Input: part model. Units: mm. Frame: model coordinates. Give positions to 0.01 mm unless a question says otherwise; leave off trailing zeros. Write each loop counter-clockwise with the first axis right and the second up, starting at its lowest first coordinate (ties: lowest second). Pieces come first, ordered by that corner, then holes. Notation, with made-up numbers: (88, 33.25) -> (98, 33.25) arc R35 ccw to (98, 72.25) -> close; hole circle Ø11 at (-23.75, 87). An arc over 180 degrees is marked (long way). Return JSON: item names as keys, results as strings. Group by question number.
Item 1: Pin query (flat end, axial travel): P1, Ø2, axis at y = 26.5, z = 5.5, coming from the +X side; P2, Ø3.5, axis at x = -30, y = -11.25, coming from the -Z side; P3, Ø2.5, axis at x = 110, y = 18.63, coming from the -Z side; P4, Ø5, axis at x = 20, y = -11.25, coming from the +Z side. Return the tip coordinate at first contact, or that it passes through.
Item 2: Section A-A, the plane x = -71. Return loops of the section in (y, z).
Item 3: Line query: line 1 (Y direction, x = 110, z = 2.5); line 2 (Y direction, x = 25, z = 2.3); line 3 (Y direction, x = -30, z = 1.35). Output: solid intervals per line, ascending. Write a range as [from, to].
from build123d import *

# Parameters (mm, degrees)
SKETCH_1_R      = 1.55
SKETCH_1_R_2    = 1.6
SKETCH_1_R_3    = 1.546583653
SKETCH_1_R_4    = 2
EXTRUDE_1_DEPTH = 4
EXTRUDE_2_DEPTH = 2


with BuildPart() as part:
    # 草图1 → 凸台-拉伸1 (new body)
    with BuildSketch(Plane.XY):
        with BuildLine():
            Line((-93.257786629, 4.43161967), (-67.403754616, 4.43161967))
            ThreePointArc((-67.403754616, 4.43161967), (-63.86822071, 2.967153575), (-62.403754616, -0.56838033))
            Line((-62.403754616, -0.56838033), (-62.403754616, -2.789641507))
            ThreePointArc((-62.403754616, -2.789641507), (-58.770779001, -11.560420508), (-50, -15.193396123))
            Line((-50, -15.193396123), (-25.75, -15.193396123))
            ThreePointArc((-25.75, -15.193396123), (-18.678932188, -18.122328311), (-15.75, -25.193396123))
            Line((-15.75, -25.193396123), (-15.75, -53.504719017))
            Line((-15.75, -53.504719017), (15.75, -53.504719017))
            Line((15.75, -53.504719017), (15.75, -25.193396123))
            ThreePointArc((15.75, -25.193396123), (18.678932188, -18.122328311), (25.75, -15.193396123))
            Line((25.75, -15.193396123), (50, -15.193396123))
            ThreePointArc((50, -15.193396123), (58.770779001, -11.560420508), (62.403754616, -2.789641507))
            Line((62.403754616, -2.789641507), (62.403754616, -0.56838033))
            ThreePointArc((62.403754616, -0.56838033), (63.86822071, 2.967153575), (67.403754616, 4.43161967))
            Line((67.403754616, 4.43161967), (93.257786629, 4.43161967))
            Line((93.257786629, 4.43161967), (115, 4.43161967))
            ThreePointArc((115, 4.43161967), (122.071067812, 7.360551858), (125, 14.43161967))
            Line((125, 14.43161967), (125, 44.220324858))
            ThreePointArc((125, 44.220324858), (122.071067812, 51.29139267), (115, 54.220324858))
            Line((115, 54.220324858), (95.550812853, 54.220324858))
            Line((95.550812853, 54.220324858), (-95.550812853, 54.220324858))
            Line((-95.550812853, 54.220324858), (-115, 54.220324858))
            ThreePointArc((-115, 54.220324858), (-122.071067812, 51.29139267), (-125, 44.220324858))
            Line((-125, 44.220324858), (-125, 14.43161967))
            ThreePointArc((-125, 14.43161967), (-122.071067812, 7.360551858), (-115, 4.43161967))
            Line((-115, 4.43161967), (-93.257786629, 4.43161967))
        make_face()
        with Locations((-10.5, -32.252284296)):
            Circle(SKETCH_1_R, mode=Mode.SUBTRACT)
        with Locations((-49, -5.252284296)):
            Circle(SKETCH_1_R, mode=Mode.SUBTRACT)
        with Locations((-30, -11.252284296)):
            Circle(SKETCH_1_R, mode=Mode.SUBTRACT)
        with Locations((-20, -11.252284296)):
            Circle(SKETCH_1_R, mode=Mode.SUBTRACT)
        with Locations((-10.5, -11.252284296)):
            Circle(SKETCH_1_R, mode=Mode.SUBTRACT)
        with Locations((-25, -0.752284296)):
            Circle(SKETCH_1_R, mode=Mode.SUBTRACT)
        with Locations((0, -42.752284296)):
            Circle(SKETCH_1_R_2, mode=Mode.SUBTRACT)
        with Locations((10.5, -32.252284296)):
            Circle(SKETCH_1_R, mode=Mode.SUBTRACT)
        with Locations((0, -21.748867949)):
            Circle(SKETCH_1_R_3, mode=Mode.SUBTRACT)
        with Locations((10.5, -11.252284296)):
            Circle(SKETCH_1_R, mode=Mode.SUBTRACT)
        with Locations((20, -11.252284296)):
            Circle(SKETCH_1_R, mode=Mode.SUBTRACT)
        with Locations((30, -11.252284296)):
            Circle(SKETCH_1_R, mode=Mode.SUBTRACT)
        with Locations((0, -0.752284296)):
            Circle(SKETCH_1_R, mode=Mode.SUBTRACT)
        with Locations((25, -0.752284296)):
            Circle(SKETCH_1_R, mode=Mode.SUBTRACT)
        with Locations((49, -5.252284296)):
            Circle(SKETCH_1_R, mode=Mode.SUBTRACT)
        with Locations((-110, 18.626388225)):
            Circle(SKETCH_1_R_4, mode=Mode.SUBTRACT)
        with BuildLine():
            ThreePointArc((-47.619318323, 12.788573549), (-49.619318323, 14.788573549), (-47.619318323, 16.788573549))
            Line((-47.619318323, 16.788573549), (-22.619318323, 16.788573549))
            ThreePointArc((-22.619318323, 16.788573549), (-20.619318323, 14.788573549), (-22.619318323, 12.788573549))
            Line((-22.619318323, 12.788573549), (-47.619318323, 12.788573549))
        make_face(mode=Mode.SUBTRACT)
        with Locations((-120.5, 29.126388225)):
            Circle(SKETCH_1_R_4, mode=Mode.SUBTRACT)
        with Locations((-99.5, 29.126388225)):
            Circle(SKETCH_1_R_4, mode=Mode.SUBTRACT)
        with Locations((-110, 39.626388225)):
            Circle(SKETCH_1_R_4, mode=Mode.SUBTRACT)
        with BuildLine():
            ThreePointArc((-47.619318323, 32.223901574), (-49.619318323, 34.223901574), (-47.619318323, 36.223901574))
            Line((-47.619318323, 36.223901574), (-22.619318323, 36.223901574))
            ThreePointArc((-22.619318323, 36.223901574), (-20.619318323, 34.223901574), (-22.619318323, 32.223901574))
            Line((-22.619318323, 32.223901574), (-47.619318323, 32.223901574))
        make_face(mode=Mode.SUBTRACT)
        with BuildLine():
            Line((22.619318323, 16.788573549), (47.619318323, 16.788573549))
            ThreePointArc((47.619318323, 16.788573549), (49.619318323, 14.788573549), (47.619318323, 12.788573549))
            Line((47.619318323, 12.788573549), (22.619318323, 12.788573549))
            ThreePointArc((22.619318323, 12.788573549), (20.619318323, 14.788573549), (22.619318323, 16.788573549))
        make_face(mode=Mode.SUBTRACT)
        with Locations((110, 18.626388225)):
            Circle(SKETCH_1_R_4, mode=Mode.SUBTRACT)
        with BuildLine():
            Line((22.619318323, 36.223901574), (47.619318323, 36.223901574))
            ThreePointArc((47.619318323, 36.223901574), (49.619318323, 34.223901574), (47.619318323, 32.223901574))
            Line((47.619318323, 32.223901574), (22.619318323, 32.223901574))
            ThreePointArc((22.619318323, 32.223901574), (20.619318323, 34.223901574), (22.619318323, 36.223901574))
        make_face(mode=Mode.SUBTRACT)
        with Locations((99.5, 29.126388225)):
            Circle(SKETCH_1_R_4, mode=Mode.SUBTRACT)
        with Locations((120.5, 29.126388225)):
            Circle(SKETCH_1_R_4, mode=Mode.SUBTRACT)
        with Locations((110, 39.626388225)):
            Circle(SKETCH_1_R_4, mode=Mode.SUBTRACT)
    extrude(amount=EXTRUDE_1_DEPTH)

    # 草图2 → 凸台-拉伸2 (add)
    with BuildSketch(Plane.XY.offset(4)):
        Polygon((3.098482938, -35.658654768), (-3.098482938, -35.658654768), (-3.098482938, 24.781778974), (-87.869942148, 24.781778974), (-87.869942148, 31.693824975), (-3.098482938, 31.693824975), (-3.098482938, 54.220324858), (3.098482938, 54.220324858), (3.098482938, 31.693824975), (87.869942148, 31.693824975), (87.869942148, 24.781778974), (3.098482938, 24.781778974), align=None)
    extrude(amount=EXTRUDE_2_DEPTH)


solid = part.part
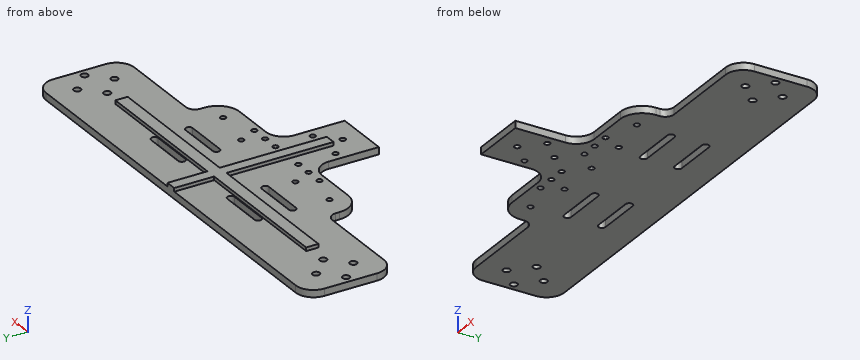
Answer below:
{
 "1": {"P1": "stops at x = 87.87", "P2": "stops at z = 0", "P3": "passes through", "P4": "stops at z = 4"},
 "2": {"outline": "(4.43, 0) -> (54.22, 0) -> (54.22, 4) -> (31.69, 4) -> (31.69, 6) -> (24.78, 6) -> (24.78, 4) -> (4.43, 4) -> close"},
 "3": {"line 1": "y = [4.43, 16.63], [20.63, 37.63], [41.63, 54.22]", "line 2": "y = [-15.22, -2.3], [0.8, 12.79], [16.79, 32.22], [36.22, 54.22]", "line 3": "y = [-15.19, -12.8], [-9.7, 12.79], [16.79, 32.22], [36.22, 54.22]"}
}
